```python
from build123d import *

# Parameters (mm, degrees)
SKETCH15_R              = 1.75
BOSS_EXTRUDE2_DEPTH     = 2
CUT_EXTRUDE1_DEPTH      = 13.136675822
CUT_EXTRUDE1_DEPTH_BACK = 13.136675822
SKETCH16_R              = 37


with BuildPart() as part:
    # Sketch15 → Boss-Extrude2 (new body)
    with BuildSketch(Plane.XY):
        Polygon((-9.33, 5.01), (-9.33, -7.5), (5, -2.5), (5, 2.5), align=None)
        Circle(SKETCH15_R, mode=Mode.SUBTRACT)
    extrude(amount=BOSS_EXTRUDE2_DEPTH)

    # Sketch16 → Cut-Extrude1 (cut, two sides: drawn at the far end of the back side and taken through both)
    with BuildSketch(Plane(origin=(0, 0, 0), x_dir=(1, 0, 0), z_dir=(0, 1, 0)).offset(-CUT_EXTRUDE1_DEPTH_BACK)):
        with Locations((-44.33, 10)):
            Circle(SKETCH16_R)
    extrude(amount=CUT_EXTRUDE1_DEPTH + CUT_EXTRUDE1_DEPTH_BACK, mode=Mode.SUBTRACT)


solid = part.part
```
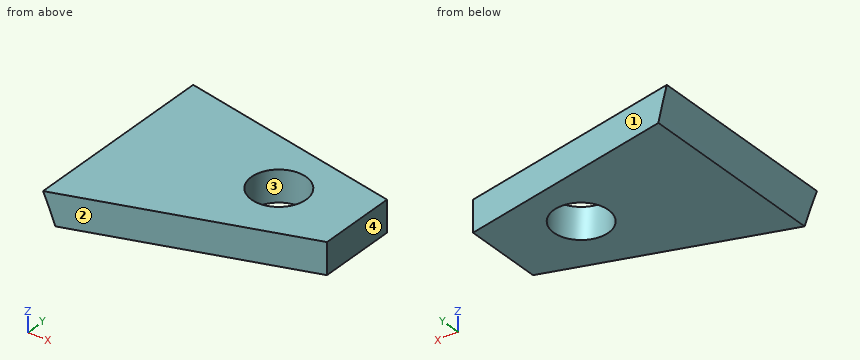
Check sheet for the modelled part. Datum: model origin and axes. Units: mm. Face numbers are marked on the shaded views. Coordinates: 2 decimals unless noted, no trailing zeros. Write each loop counter-clockwise with the first axis right and the second up, starting at its lowest first coordinate (ties: lowest second). Pieces come first, ordered by that corner, then holes. Notation, with made-up numbers: (82, 27) -> (95, 27) arc R10 cw to (95, 41) -> close; hole circle Ø1 at (-0.5, 15). An arc over 180 degrees is marked (long way). Use a Markdown table: item, result.
1. Sectioned sample at A-A (y = 0). Enter the section's corners in (x, z), plus the area to 3 significant figures.
Reported:
| item | result |
|---|---|
| outline | (-9.33, 2) arc R37 cw to (-8.71, 0) -> (-1.75, 0) -> (-1.75, 2) -> close; (1.75, 0) -> (5, 0) -> (5, 2) -> (1.75, 2) -> close |
| area | 21.0 mm2 |
2. Sectioned sample at D-D (x = -4). Enter the section's corners in (y, z), plus the area to 3 significant figures.
Reported:
| item | result |
|---|---|
| outline | (-5.64, 0) -> (4.08, 0) -> (4.08, 2) -> (-5.64, 2) -> close |
| area | 19.4 mm2 |
3. Sectioned sample at C-C (z = 1.75). Enter the section's corners in (x, y), plus the area to 3 significant figures.
Reported:
| item | result |
|---|---|
| outline | (-9.25, -7.47) -> (5, -2.5) -> (5, 2.5) -> (-9.25, 5) -> close; hole circle Ø3.5 at (0, 0) |
| area | 115 mm2 |
4. Go/stop test with a flat-tipped pin: pin 1 Ø4 at (x, y) = (0, 0) entering from -Z. Record where the tip stops, or that it passes through.
Reported:
| item | result |
|---|---|
| pin 1 | stops at z = 0 |
5. Release check for a two-part mould opening along Y. For the marked faces 1, 2, 3 and 4 record: pulls with the +Y half, pulls with the -Y half, needs draft (parallel to the pull), parting line crosses it, or undercut.
Reported:
| item | result |
|---|---|
| face 1 | pulls with the +Y half |
| face 2 | pulls with the -Y half |
| face 3 | undercut |
| face 4 | needs draft |
6. Scan lines: line 1 along Y through (x, z) = (0, 1.1); line 2 along X through (y, z) = (-0.5, 1.1); line 3 along Y through (x, z) = (0.75, 1.75). Record each from-to range of solid material in increasing order.
Reported:
| item | result |
|---|---|
| line 1 | y = -4.24 to -1.75, 1.75 to 3.38 |
| line 2 | x = -9.03 to -1.68, 1.68 to 5 |
| line 3 | y = -3.98 to -1.58, 1.58 to 3.24 |
7. Sectioned sample at B-B (x = -1.5). Enter the section's corners in (y, z), plus the area to 3 significant figures.
Reported:
| item | result |
|---|---|
| outline | (-4.77, 0) -> (-0.9, 0) -> (-0.9, 2) -> (-4.77, 2) -> close; (0.9, 0) -> (3.64, 0) -> (3.64, 2) -> (0.9, 2) -> close |
| area | 13.2 mm2 |
